from build123d import *

# Parameters (mm, degrees)
SKETCH1_R           = 10
BOSS_EXTRUDE1_DEPTH = 10
SKETCH2_R           = 7.5
BOSS_EXTRUDE2_DEPTH = 30
SKETCH3_R           = 10
BOSS_EXTRUDE3_DEPTH = 10
SKETCH4_R           = 7.5
BOSS_EXTRUDE4_DEPTH = 30


with BuildPart() as part:
    # Sketch1 → Boss-Extrude1 (new body, symmetric)
    with BuildSketch(Plane.XY):
        Circle(SKETCH1_R)
    extrude(amount=BOSS_EXTRUDE1_DEPTH, both=True)

    # Sketch2 → Boss-Extrude2 (add, symmetric)
    with BuildSketch(Plane.XY):
        Circle(SKETCH2_R)
    extrude(amount=BOSS_EXTRUDE2_DEPTH, both=True)

    # Sketch3 → Boss-Extrude3 (add, symmetric)
    with BuildSketch(Plane(origin=(0, 0, 0), x_dir=(1, 0, 0), z_dir=(0, 1, 0))):
        Circle(SKETCH3_R)
    extrude(amount=BOSS_EXTRUDE3_DEPTH, both=True)

    # Sketch4 → Boss-Extrude4 (add, symmetric)
    with BuildSketch(Plane(origin=(0, 0, 0), x_dir=(1, 0, 0), z_dir=(0, 1, 0))):
        Circle(SKETCH4_R)
    extrude(amount=BOSS_EXTRUDE4_DEPTH, both=True)


solid = part.part
The listing builds one solid part. Answer for the finished solid, in the listing's coordinates (mm). A direction names the side the tool comes from. Round coordinates to 2 decimals unless told otherwise and drop trailing zeros. Order: outer loops, then holes, each group sorted by start corner. A loop starts at its lowest first (then second) coordinate and runs counter-clockwise, first axis right, second up. Notation, with made-up numbers: M -6.75,-21.5 L 46.25,-21.5 A29 cw 46.25,12.5 Z; hole C -36.5,-3.5 d10. An arc over 180 degrees is marked long. Answer in a Markdown table with one row per item. Add a question column.
1) The part is cut by section D-D on x = 8.25. Determine the outline of the cut face in (y, z), plus the area to 3 significant figures.
2) Consider line 1 along Y through (x, z) = (-0.5, 27); line 2 along Y through (x, z) = (-3, -9). Determine where each line is inside the solid, lowest interval first. Write a range as from..to.
3) The part is cut by section B-B on z = -25. Determine the outline of the cut face in (x, y), plus the area to 3 significant figures.
4) The part is cut by section A-A on x = -2. Determine the outline of the cut face in (y, z).
5) Which of the six approach directions +Z, -Z, +X, -X, +Y, -Y give full straight-line access (tool end or side, diameter ignored) to faces 1 (the face through (4, 7, -10)), 2 (the face through (-7.493, 20.14, -0.33)), 3 (the face through (10, -6, 0))?
6) Flat-ended cylindrical pins translate along their axes: pin 1 Ø1 at (y, z) = (19, 0.5) entering from +X; pin 2 Ø1.5 at (y, z) = (-6.5, -18) entering from -X; pin 3 Ø4 at (x, y) = (7.5, 18) entering from +Z; pin 4 Ø12 at (y, z) = (8, -5.5) entering from -X. Find the tip coordinate at first contact, or state that the pin passes through.
Findings below:
| question | item | result |
|---|---|---|
| 1 | outline | M -10,-5.65 L -5.65,-5.65 L -5.65,-10 L 5.65,-10 L 5.65,-5.65 L 10,-5.65 L 10,5.65 L 5.65,5.65 L 5.65,10 L -5.65,10 L -5.65,5.65 L -10,5.65 Z |
| 1 | area | 324 mm² |
| 2 | line 1 | y = -7.48..7.48 |
| 2 | line 2 | y = -10..10 |
| 3 | outline | C 0,0 d15 |
| 3 | area | 177 mm² |
| 4 | outline | M -30,-7.23 L -10,-7.23 L -10,-9.8 L -9.8,-9.8 L -9.8,-10 L -7.23,-10 L -7.23,-30 L 7.23,-30 L 7.23,-10 L 9.8,-10 L 9.8,-9.8 L 10,-9.8 L 10,-7.23 L 30,-7.23 L 30,7.23 L 10,7.23 L 10,9.8 L 9.8,9.8 L 9.8,10 L 7.23,10 L 7.23,30 L -7.23,30 L -7.23,10 L -9.8,10 L -9.8,9.8 L -10,9.8 L -10,7.23 L -30,7.23 Z |
| 5 | face 1 | -Z |
| 5 | face 2 | +Y |
| 5 | face 3 | +X, -Y |
| 6 | pin 1 | stops at x = 7.5 |
| 6 | pin 2 | stops at x = -4.82 |
| 6 | pin 3 | stops at z = 5.1 |
| 6 | pin 4 | stops at x = -10 |
